from build123d import *

# Parameters (mm, degrees)
F0_R     = 6.35
F1_DEPTH = 12.7
F3_DEPTH = 12.7
F4_W     = 25.4
F4_H     = 31.75
F4_H_2   = 12.7
F5_DEPTH = 12.7
F7_DEPTH = 12.7
F9_DEPTH = 12.7


with BuildPart() as f1:
    # F0 (on Top) → F1 (new body)
    with BuildSketch(Plane.XY):
        with BuildLine():
            Line((31.75, 25.4), (0, 25.4))
            Line((0, 25.4), (0, 0))
            Line((0, 0), (31.75, 0))
            ThreePointArc((31.75, 0), (44.304303, 12.7), (31.75, 25.4))
        make_face()
        with Locations((12.7, 12.7)):
            Circle(F0_R, mode=Mode.SUBTRACT)
        with Locations((31.75, 12.7)):
            Circle(F0_R, mode=Mode.SUBTRACT)
        with BuildLine():
            Line((44.45, 25.4), (31.75, 25.4))
            ThreePointArc((31.75, 25.4), (44.304303, 12.7), (31.75, 0))
            Line((31.75, 0), (44.45, 0))
            Line((44.45, 0), (44.45, 25.4))
        make_face()
    extrude(amount=F1_DEPTH)

    # F2 (on face) → F3 (cut)
    with BuildSketch(Plane.XY.offset(12.7)):
        with BuildLine():
            ThreePointArc((31.866888, 25.4), (44.112876, 12.548889), (31.557373, 0))
            Line((31.557373, 0), (44.45, 0))
            Line((44.45, 0), (44.45, 25.4))
            Line((44.45, 25.4), (31.866888, 25.4))
        make_face()
    extrude(amount=-F3_DEPTH, mode=Mode.SUBTRACT)

    # F4 (on face) → F5 (join)
    with BuildSketch(Plane(origin=(0, 0, 0), x_dir=(0, -1, 0), z_dir=(-1, 0, 0))):
        with Locations((-12.7, 28.575)):
            Rectangle(F4_W, F4_H)
        with Locations((-12.7, 6.35)):
            Rectangle(F4_W, F4_H_2)
    extrude(amount=F5_DEPTH)

    # F6 (on face) → F7 (cut)
    with BuildSketch(Plane(origin=(-12.7, 0, 0), x_dir=(0, -1, 0), z_dir=(-1, 0, 0))):
        with BuildLine():
            Line((-6.35, 44.45), (-19.05, 44.45))
            Line((-19.05, 44.45), (-19.05, 31.75))
            ThreePointArc((-19.05, 31.75), (-12.7, 25.4), (-6.35, 31.75))
            Line((-6.35, 31.75), (-6.35, 44.45))
        make_face()
    extrude(amount=-F7_DEPTH, mode=Mode.SUBTRACT)

    # F8 (on face) → F9 (cut)
    with BuildSketch(Plane(origin=(-12.7, 0, 0), x_dir=(0, -1, 0), z_dir=(-1, 0, 0))):
        with BuildLine():
            ThreePointArc((-25.4, 31.75), (-23.698523, 38.1), (-19.05, 42.748523))
            Line((-19.05, 42.748523), (-19.05, 44.45))
            Line((-19.05, 44.45), (-25.4, 44.45))
            Line((-25.4, 44.45), (-25.4, 31.75))
        make_face()
        with BuildLine():
            ThreePointArc((-6.35, 42.748523), (-1.701477, 38.1), (0, 31.75))
            Line((0, 31.75), (0, 44.45))
            Line((0, 44.45), (-6.35, 44.45))
            Line((-6.35, 44.45), (-6.35, 42.748523))
        make_face()
    extrude(amount=-F9_DEPTH, mode=Mode.SUBTRACT)


solid = f1.part
Source: CAD feature listing. Evaluate the final solid. Frame: model axes, mm. A direction names the side the tool comes from. Round coordinates to 2 decimals unless told otherwise and drop trailing zeros. Write each loop counter-clockwise with the first axis right and the second up, starting at its lowest first coordinate (ties: lowest second). Pieces come first, ordered by that corner, then holes. Notation, with made-up numbers: (-20.5, 59) - (0.5, 59) arc R20 cw to (0.5, 98) - close; hole circle Ø7 at (-26, 60.25). An arc over 180 degrees is marked (long way). Use CSV: the item, a comma, the result in double quotes. Start each with the question number.
(1) Cut plane D-D, the plane y = 16. Return loops of the section in (x, z).
(2) Set-up query: faces 4 (the face through (0, 13, 25)), 5 (the face through (8.02, 16.99, 6.26)), 6 (the face through (-6, 6.35, 37)). Return all of +Z, -Z, +X, -X, +Y, -Y with unobstructed straight access to the full face (end or side cutting, diameter ignored); none if empty.
(3) Cut plane C-C, the plane z = 29.5. Return loops of the section in (x, y).
(4) Mould query, pull axis Y, two halves, no side actions, for faces 1 (the face through (35.164, 18.054, 6.261)), 2 (the face through (5, 0, 12)), 3 (the face through (-6.439, 23.745, 38.019)). Classes: pulls with the +Y half, pulls with the -Y half, needs draft (parallel to the pull), parting line crosses it, or undercut.
(5) Cut plane A-A, the plane y = 12.7. Return loops of the section in (x, z), and give its area (3 significant figures).
(6) Cut plane B-B, the plane x = 12.7. Return loops of the section in (y, z), and give its area (3 significant figures).
(7) First-contact query: pin 1 Ø10 at (y, z) = (21, 24) entering from +X; pin 2 Ø3 at (x, y) = (38, 21.5) entering from +Z; pin 3 Ø3.5 at (x, z) = (-6.5, 34.5) entering from +Y. Flat tips, straight axial feed; report the tip coordinate or a pass-through.
(8) Material intervals for probe 1 along Y at (x, z) = (31.75, 7); probe 2 along X at (y, z) = (7.25, 17); probe 3 along Z at (x, y) = (28, 3.75), sorted ascending. Write a range as [from, to].
Geometry says:
1,outline,"(-12.7, 0) - (7.27, 0) - (7.27, 12.7) - (0, 12.7) - (0, 26.32) - (-12.7, 26.32) - close; (18.13, 0) - (26.32, 0) - (26.32, 12.7) - (18.13, 12.7) - close; (37.18, 0) - (43.68, 0) - (43.68, 12.7) - (37.18, 12.7) - close"
2,face 4,"+Z, +X, +Y, -Y"
2,face 5,"+Z, -Z"
2,face 6,"+Z, +X, -X"
3,outline,"(-12.7, 0) - (0, 0) - (0, 6.76) - (-12.7, 6.76) - close; (-12.7, 18.64) - (0, 18.64) - (0, 25.4) - (-12.7, 25.4) - close"
4,face 1,"undercut"
4,face 2,"pulls with the -Y half"
4,face 3,"pulls with the +Y half"
5,outline,"(-12.7, 0) - (6.35, 0) - (6.35, 12.7) - (0, 12.7) - (0, 25.4) - (-12.7, 25.4) - close; (19.05, 0) - (25.4, 0) - (25.4, 12.7) - (19.05, 12.7) - close; (38.1, 0) - (44.11, 0) - (44.11, 12.7) - (38.1, 12.7) - close"
5,area,"560 mm²"
6,outline,"(0, 0) - (6.35, 0) - (6.35, 12.7) - (0, 12.7) - close; (19.05, 0) - (25.4, 0) - (25.4, 12.7) - (19.05, 12.7) - close"
6,area,"161 mm²"
7,pin 1,"x = 0"
7,pin 2,"z = 12.7"
7,pin 3,"y = 25.36"
8,probe 1,"[0, 6.35], [19.05, 25.4]"
8,probe 2,"[-12.7, 0]"
8,probe 3,"[0, 12.7]"
